Geometry check sheet. Reference: drawing and pictorial views, mm from the part's lowest x, y, z. A direction names the side the tool comes from. Round coordinates to 2 decimals unless told otherwise and drop trailing zeros. Loops run counter-clockwise (first coordinate to the right, second up) from the corner with the lowest first, then second, coordinate; pieces in that order, holes last. Notation, with made-up numbers: (-11, 20.25) - (-5, 20.25) arc R27 cw to (-5, 55.25) - close; hole circle Ø9 at (23, -15.75). An arc over 180 degrees is marked (long way). Put each result on its own line as item: value. Start each with the question number.
Item 1: Section check A-A, the plane z = 10. Record the cut outline in (x, y) (1 decimal).
Item 2: Section check C-C, the plane y = 9.25. Record the cut outline in (x, z) (1 decimal), and give its area (3 significant figures).
Item 3: Section check B-B, the plane x = 6. Record the cut outline in (y, z) (1 decimal).
Item 4: Section check D-D, the plane x = 1.5. Record the cut outline in (y, z).
Item 5: Draft check along Y on the marked faces 1, 2 and 3. Enter one of: pulls with the +Y half, pulls with the -Y half, needs draft (parallel to the pull), parting line crosses it, or undercut.
Item 6: Tool access check on the marked faces 4 and 5. Record the directions out of +Z, -Z, +X, -X, +Y, -Y that give a thin tool (end or side, any length) a straight path to the whole face; none if there is none.
Item 7: Gauge pin test, flat ends, axial feed: pin 1 Ø1.5 at (x, z) = (3, 61) entering from -Y; pin 2 Ø1.5 at (x, y) = (8, 2.5) entering from -Z; pin 3 Ø5.5 at (x, y) = (6.5, 10.5) entering from -Z; pin 4 Ø5 at (x, y) = (4, 16) entering from +Z. Record the tip position at first contact, or that the pin passes through.
Item 8: Material ranges on line 1 along Y through (x, z) = (6, 15); line 2 along X through (y, z) = (4.05, 10) (1 decimal); line 3 along Z through (x, y) = (5.5, 3), recorded low to high.
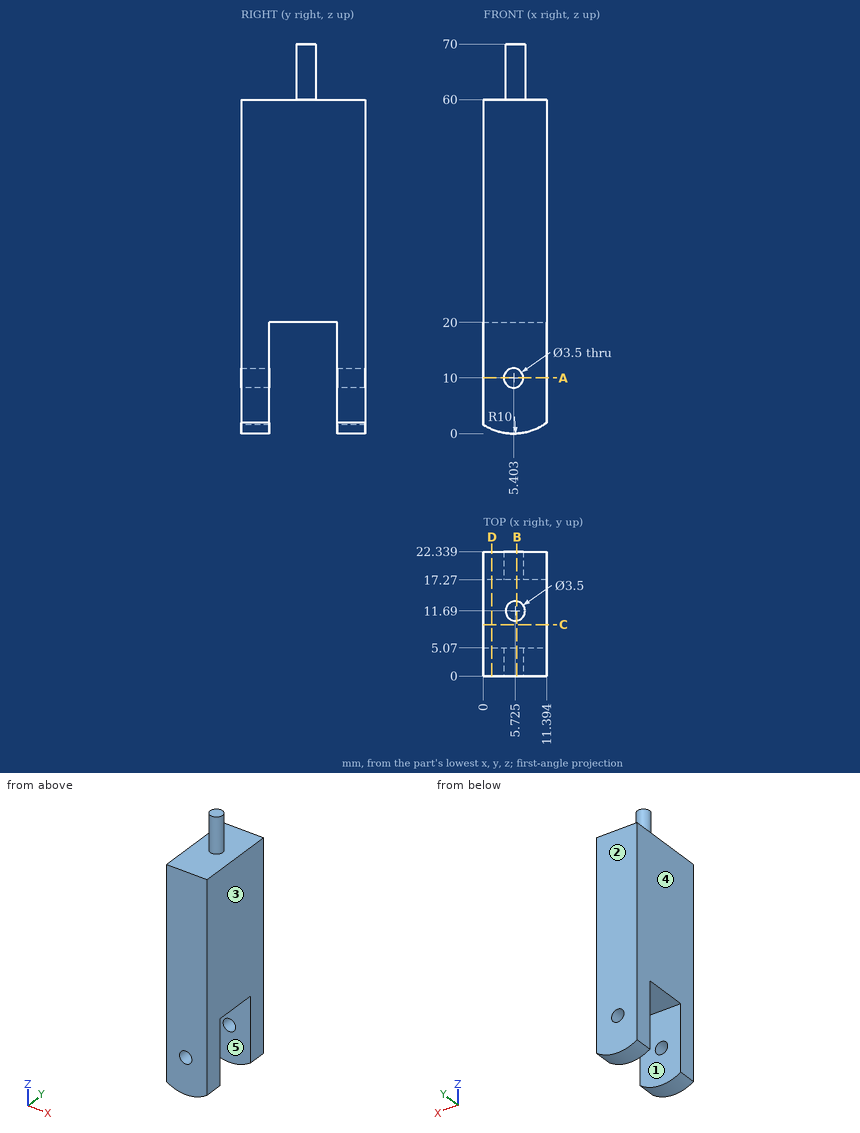
Check result:
1. outline: (0, 0) - (3.7, 0) - (3.7, 5.1) - (0, 5.1) - close; (0, 17.3) - (3.7, 17.3) - (3.7, 22.3) - (0, 22.3) - close; (7.2, 0) - (11.4, 0) - (11.4, 5.1) - (7.2, 5.1) - close; (7.2, 17.3) - (11.4, 17.3) - (11.4, 22.3) - (7.2, 22.3) - close
2. outline: (0, 20) - (11.4, 20) - (11.4, 60) - (0, 60) - close
2. area: 456 mm²
3. outline: (0, 0) - (5.1, 0) - (5.1, 8.4) - (0, 8.4) - close; (0, 11.6) - (5.1, 11.6) - (5.1, 20) - (17.3, 20) - (17.3, 11.6) - (22.3, 11.6) - (22.3, 60) - (13.4, 60) - (13.4, 70) - (10, 70) - (10, 60) - (0, 60) - close; (17.3, 0) - (22.3, 0) - (22.3, 8.4) - (17.3, 8.4) - close
4. outline: (0, 0.79) - (5.07, 0.79) - (5.07, 20) - (17.27, 20) - (17.27, 0.79) - (22.34, 0.79) - (22.34, 60) - (0, 60) - close
5. face 1: undercut
5. face 2: pulls with the +Y half
5. face 3: needs draft
6. face 4: +Z, -Z, -X, +Y, -Y
6. face 5: -Z, +X, -X
7. pin 1: through
7. pin 2: z = 0.17
7. pin 3: z = 20
7. pin 4: z = 60
8. line 1: 0 to 5.07, 17.27 to 22.34
8. line 2: 0 to 3.7, 7.2 to 11.4
8. line 3: 0 to 8.25, 11.75 to 60
